Can you work these out from the model? Positions are in its coordinate system, mm. Face numbers are marked on the shaded views. A direction names the side the tool comes from. Coordinates: 2 decimals unless noted, no trailing zeros. Order: outer loops, then holes, each group sorted by start corner. A loop starts at its lowest first (then second) coordinate and runs counter-clockwise, first axis right, second up. Notation, with made-up numbers: (-9.5, 0.5) -> (26.5, 0.5) arc R17 cw to (26.5, 12.5) -> close; hole circle Ø10 at (40.25, 9.25). An arc over 180 degrees is marked (long way). Answer as a JSON object with one key per item and string values. Group by question number.
(1) I want a section at B-B, the plane z = 3. List the corners of the cut face in (x, y) for me.
(2) I want a section at D-D, the plane y = 0. List the corners of the cut face in (x, z) for me.
(3) I want a section at A-A, the plane y = -40. List the corners of the cut face in (x, z) for me.
(4) I want a section at C-C, the plane x = -5.15. List the corners of the cut face in (y, z) for me, plus the area to 3 significant figures.
(5) If we mould it in two halves opening along Y, with no side actions, what happens to the marked faces 1, 2, 3 and 4? For each: pulls with the +Y half, pulls with the -Y half, needs draft (parallel to the pull), parting line crosses it, or undercut.
(6) Which directions (+Z, -Z, +X, -X, +Y, -Y) give clear straight access to the entire face, cutting with the end or side of a thin tool? Please do the marked faces 5 and 6.
(7) For pin 1 (10 mm diameter, centred on x = -17, z = 38, fed in from -Y); pin 2 (4 mm diameter, centred on x = -15, z = 7.25, fed in from -Y); pin 3 (4 mm diameter, centred on y = -40, z = 3, fed in from -X); pin 4 (2 mm diameter, centred on y = 7.5, z = 11, fed in from +X), each with a flat end and sliding along its axis, tell me the tip position at first contact or that it passes through.
(8) I need wall thicknesses on line 1 (Y direction, x = -38.5, z = 32); line 2 (Z direction, x = -12, y = 40); line 3 (X direction, y = -47.85, z = 7.25) (3 decimals). Which ranges of each line are inside material? Lowest first, please.
from build123d import *

# Parameters (mm, degrees)
CENTRE_HOLE_FOR_L2_DEPTH      = 40
CENTRE_HOLE_FOR_L2_DEPTH_BACK = 10
SKETCH1_R                     = 39.1
SKETCH1_R_2                   = 31.75
MAIN_STRUCTURE_DEPTH          = 60
MAIN_STRUCTURE_DEPTH_BACK     = 50
SKETCH2_W                     = 100
SKETCH2_H                     = 100
SKETCH2_R                     = 39.1
BEARING_CURVE_DEPTH           = 10
SKETCH6_R                     = 10.5
SHAFT_HOLE_DEPTH              = 10
WRIST_CUTOUT_DEPTH            = 188.082869339
SKETCH11_W                    = 25
SKETCH11_H                    = 45
SKETCH11_R                    = 2.525
BOSS_EXTRUDE1_DEPTH           = 6
SKETCH15_W                    = 19.8
SKETCH15_H                    = 7
CUT_EXTRUDE4_DEPTH            = 4
CUT_EXTRUDE5_REACH            = 190.16
CUT_EXTRUDE5_END_RADIUS       = 31.75
SKETCH16_R                    = 1.5
CUT_EXTRUDE6_DEPTH            = 168.7378908
CUT_EXTRUDE6_DEPTH_BACK       = 168.7378908
SKETCH18_R                    = 3.25
CUT_EXTRUDE7_START            = -1.5875
CUT_EXTRUDE7_DEPTH            = 1.5875
SKETCH9_R                     = 12.05
BEARING_DEPTH                 = 5
CUT_EXTRUDE8_DEPTH            = 3
SKETCH21_R                    = 3.25
SKETCH21_R_2                  = 1.65
CUT_EXTRUDE9_DEPTH            = 167.868211501
CUT_EXTRUDE10_DEPTH           = 6.35
SKETCH23_R                    = 2.275
CUT_EXTRUDE11_DEPTH           = 6
CHAMFER1_SIZE                 = 0.5


with BuildPart() as part:
    # Sketch1 → Centre Hole for L2 (new, two sides: drawn at the far end of the back side and taken through both)
    with BuildSketch(Plane.XY.offset(-CENTRE_HOLE_FOR_L2_DEPTH_BACK)):
        Circle(SKETCH1_R)
        Circle(SKETCH1_R_2, mode=Mode.SUBTRACT)
    extrude(amount=CENTRE_HOLE_FOR_L2_DEPTH + CENTRE_HOLE_FOR_L2_DEPTH_BACK)

    # Sketch2 → Main Structure (add, two sides: drawn at the far end of the back side and taken through both)
    with BuildSketch(Plane.XY.offset(40).offset(-MAIN_STRUCTURE_DEPTH_BACK)):
        Rectangle(SKETCH2_W, SKETCH2_H)
        Circle(SKETCH2_R, mode=Mode.SUBTRACT)
    extrude(amount=MAIN_STRUCTURE_DEPTH + MAIN_STRUCTURE_DEPTH_BACK)

    # Sketch3 → Bearing Curve (add)
    with BuildSketch(Plane.ZY.offset(50)):
        with BuildLine():
            Line((100, 50), (100, -50))
            ThreePointArc((100, -50), (150, 0), (100, 50))
        make_face()
    bearing_curve = extrude(amount=-BEARING_CURVE_DEPTH)

    # Upright Mirror: Bearing Curve across plane
    add(bearing_curve.mirror(Plane(origin=(0, 0, 0), x_dir=(0, 0, 1), z_dir=(1, 0, 0))))

    # Sketch6 → Shaft Hole (cut)
    with BuildSketch(Plane.ZY.offset(50)):
        with Locations((100, 0)):
            Circle(SKETCH6_R)
    extrude(amount=-SHAFT_HOLE_DEPTH, mode=Mode.SUBTRACT)

    # Sketch4 → Wrist Cutout (cut, through all)
    with BuildSketch(Plane(origin=(0, 50, 0), x_dir=(1, 0, 0), z_dir=(0, 1, 0))):
        with BuildLine():
            Line((-40, -100), (-40, -60))
            ThreePointArc((-40, -60), (-34.142135624, -45.857864376), (-20, -40))
            Line((-20, -40), (20, -40))
            ThreePointArc((20, -40), (34.142135624, -45.857864376), (40, -60))
            Line((40, -60), (40, -100))
            Line((40, -100), (-40, -100))
        make_face()
    extrude(amount=-WRIST_CUTOUT_DEPTH, mode=Mode.SUBTRACT)

    # SurfaceCut1
    split(bisect_by=Plane.ZY, keep=Keep.TOP)

    # Sketch11 → Boss-Extrude1 (add)
    with BuildSketch(Plane(origin=(0, 50, 0), x_dir=(1, 0, 0), z_dir=(0, 1, 0))):
        with Locations((-12.5, -15)):
            Rectangle(SKETCH11_W, SKETCH11_H)
        with Locations(Location((-19, 1, 0), (0, 0, 270))):
            Circle(SKETCH11_R, mode=Mode.SUBTRACT)
        with Locations(Location((-19, -31, 0), (0, 0, 270))):
            Circle(SKETCH11_R, mode=Mode.SUBTRACT)
    extrude(amount=BOSS_EXTRUDE1_DEPTH)

    # Sketch15 → Cut-Extrude4 (cut)
    with BuildSketch(Plane(origin=(0, -50, 0), x_dir=(-1, 0, 0), z_dir=(0, -1, 0))):
        with Locations((9.9, -36.5)):
            Rectangle(SKETCH15_W, SKETCH15_H)
    extrude(amount=-CUT_EXTRUDE4_DEPTH, mode=Mode.SUBTRACT)

    # Cut-Extrude5: up to this cylinder (the profile starts outside it)
    cut_extrude5_end = Plane(origin=(0, 0, 35.9), z_dir=(0, 0, 1)) * Cylinder(CUT_EXTRUDE5_END_RADIUS, 444.82, mode=Mode.PRIVATE)
    # Sketch16 → Cut-Extrude5 (cut, up to the surface)
    with BuildSketch(Plane(origin=(0, -46, 0), x_dir=(-1, 0, 0), z_dir=(0, -1, 0)), mode=Mode.PRIVATE) as cut_extrude5_sk1:
        with Locations(Location((14.65, -35.9, 0), (0, 0, 90))):
            Circle(SKETCH16_R)
    cut_extrude5_tool1 = extrude(cut_extrude5_sk1.sketch, amount=-CUT_EXTRUDE5_REACH, mode=Mode.PRIVATE) - cut_extrude5_end
    add(cut_extrude5_tool1.solids().sort_by_distance((-14.65, -46, 35.9))[0], mode=Mode.SUBTRACT)
    # Sketch16 → Cut-Extrude5 (cut, up to the surface)
    with BuildSketch(Plane(origin=(0, -46, 0), x_dir=(-1, 0, 0), z_dir=(0, -1, 0)), mode=Mode.PRIVATE) as cut_extrude5_sk2:
        with Locations(Location((5.15, -35.9, 0), (0, 0, 90))):
            Circle(SKETCH16_R)
    cut_extrude5_tool2 = extrude(cut_extrude5_sk2.sketch, amount=-CUT_EXTRUDE5_REACH, mode=Mode.PRIVATE) - cut_extrude5_end
    add(cut_extrude5_tool2.solids().sort_by_distance((-5.15, -46, 35.9))[0], mode=Mode.SUBTRACT)

    # Sketch18 → Cut-Extrude6 (cut, two sides: drawn at the far end of the back side and taken through both)
    with BuildSketch(Plane.ZY.offset(50).offset(-CUT_EXTRUDE6_DEPTH_BACK)):
        with Locations((8, 0)):
            Circle(SKETCH18_R)
        with Locations((32, 0)):
            Circle(SKETCH18_R)
    extrude(amount=CUT_EXTRUDE6_DEPTH + CUT_EXTRUDE6_DEPTH_BACK, mode=Mode.SUBTRACT)

    # Sketch19 → Cut-Extrude7 (cut)
    with BuildSketch(Plane(origin=(-40, 0, 0), x_dir=(0, 0, -1), z_dir=(1, 0, 0)).offset(CUT_EXTRUDE7_START)):
        with BuildLine():
            Line((-60, 50), (-100, 50))
            ThreePointArc((-100, 50), (-150, 0), (-100, -50))
            Line((-100, -50), (-60, -50))
            Line((-60, -50), (-60, 50))
        make_face()
    extrude(amount=CUT_EXTRUDE7_DEPTH, mode=Mode.SUBTRACT)

    # Sketch9 → Bearing (cut)
    with BuildSketch(Plane(origin=(-41.5875, 0, 0), x_dir=(0, 0, -1), z_dir=(1, 0, 0))):
        with Locations((-100, 0)):
            Circle(SKETCH9_R)
    extrude(amount=-BEARING_DEPTH, mode=Mode.SUBTRACT)

    # Sketch20 → Cut-Extrude8 (cut)
    with BuildSketch(Plane.ZY.offset(50)):
        with BuildLine():
            Line((-10, -50), (100, -50))
            ThreePointArc((100, -50), (150, 0), (100, 50))
            Line((100, 50), (-10, 50))
            Line((-10, 50), (-10, -50))
        make_face()
    extrude(amount=-CUT_EXTRUDE8_DEPTH, mode=Mode.SUBTRACT)

    # Sketch21 → Cut-Extrude9 (cut, through all)
    with BuildSketch(Plane.ZY.offset(47)):
        with Locations((3, -40)):
            Circle(SKETCH21_R)
        with Locations((27, -40)):
            Circle(SKETCH21_R)
        with Locations(Location((27, 40, 0), (0, 0, 180))):
            Circle(SKETCH21_R)
        with Locations(Location((3, 40, 0), (0, 0, 180))):
            Circle(SKETCH21_R)
        with Locations((125, 0)):
            Circle(SKETCH21_R_2)
    extrude(amount=-CUT_EXTRUDE9_DEPTH, mode=Mode.SUBTRACT)

    # Sketch22 → Cut-Extrude10 (cut)
    with BuildSketch(Plane.ZY.offset(47)):
        with BuildLine():
            Line((-10, 50), (-10, -50))
            Line((-10, -50), (100, -50))
            ThreePointArc((100, -50), (150, 0), (100, 50))
            Line((100, 50), (-10, 50))
        make_face()
    extrude(amount=-CUT_EXTRUDE10_DEPTH, mode=Mode.SUBTRACT)

    # Sketch23 → Cut-Extrude11 (cut)
    with BuildSketch(Plane(origin=(0, -50, 0), x_dir=(-1, 0, 0), z_dir=(0, -1, 0))):
        with Locations(Location((15, -7.25, 0), (0, 0, 90))):
            Circle(SKETCH23_R)
    extrude(amount=-CUT_EXTRUDE11_DEPTH, mode=Mode.SUBTRACT)

    # Chamfer1
    chamfer1_edges = [part.edges().sort_by_distance(p)[0] for p in [
        (-15, -50, 9.525),
    ]]
    chamfer(chamfer1_edges, length=CHAMFER1_SIZE)


solid = part.part
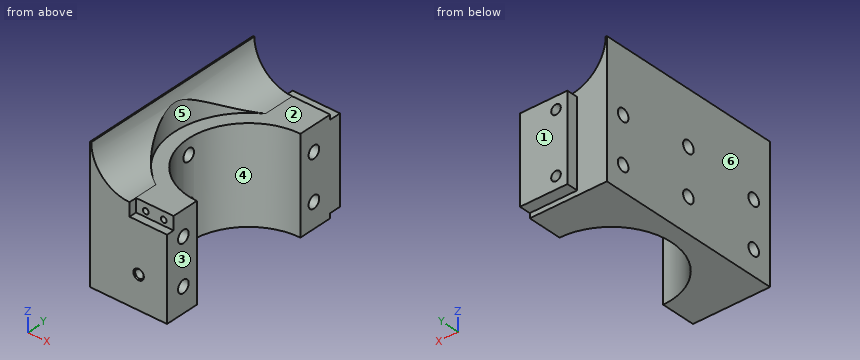
Computed values:
{
 "1": {"outline": "(-40.65, -50) -> (0, -50) -> (0, -43.25) -> (-40.65, -43.25) -> close; (-40.65, -36.75) -> (0, -36.75) -> (0, -31.75) arc R31.75 cw to (0, 31.75) -> (0, 36.75) -> (-40.65, 36.75) -> close; (-40.65, 43.25) -> (0, 43.25) -> (0, 56) -> (-25, 56) -> (-25, 50) -> (-40.65, 50) -> close"},
 "2": {"outline": "(-40.65, -10) -> (-31.75, -10) -> (-31.75, 4.75) -> (-40.65, 4.75) -> close; (-40.65, 11.25) -> (-31.75, 11.25) -> (-31.75, 28.75) -> (-40.65, 28.75) -> close; (-40.65, 35.25) -> (-31.75, 35.25) -> (-31.75, 40) -> (-39.1, 40) -> (-39.1, 54.07) arc R20 cw to (-40, 60) -> (-40.65, 60) -> close"},
 "3": {"outline": "(-40.65, -10) -> (0, -10) -> (0, -0.25) -> (-40.65, -0.25) -> close; (-40.65, 6.25) -> (0, 6.25) -> (0, 23.75) -> (-40.65, 23.75) -> close; (-40.65, 30.25) -> (0, 30.25) -> (0, 40) -> (-20, 40) arc R20 cw to (-40, 60) -> (-40.65, 60) -> close; hole circle Ø3 at (-14.65, 35.9); hole circle Ø3 at (-5.15, 35.9)"},
 "4": {"outline": "(-50, -10) -> (-31.33, -10) -> (-31.33, 34.4) -> (-46, 34.4) -> (-46, 33) -> (-50, 33) -> close; (-46, 37.4) -> (-31.33, 37.4) -> (-31.33, 40) -> (-46, 40) -> close; (31.33, -10) -> (50, -10) -> (50, -7.5) -> (56, -7.5) -> (56, 37.5) -> (50, 37.5) -> (50, 40) -> (31.33, 40) -> close; hole circle Ø6.5 at (-40, 3); hole circle Ø6.5 at (-40, 27); hole circle Ø6.5 at (40, 3); hole circle Ø6.5 at (40, 27)", "area": "1,930 mm2"},
 "5": {"face 1": "pulls with the +Y half", "face 2": "undercut", "face 3": "needs draft", "face 4": "undercut"},
 "6": {"face 5": "+Z, +X", "face 6": "+Z, -Z, -X, +Y, -Y"},
 "7": {"pin 1": "stops at y = -50", "pin 2": "stops at y = -44", "pin 3": "passes through", "pin 4": "stops at x = -30.59"},
 "8": {"line 1": "y = -50 to -3.25, 3.25 to 50", "line 2": "z = -10 to -0.25, 6.25 to 23.75, 30.25 to 40", "line 3": "x = -40.65 to -17.275, -12.725 to 0"}
}
